Can you work these out from the drawing? Everything is in mm from the part's minimum corner. A direction names the side the tool comes from. Coordinates: 2 decimals unless noted, no trailing zeros. Loops run counter-clockwise (first coordinate to the right, second up) from the corner with the lowest first, then second, coordinate; pieces in that order, holes last. Notation, with made-up numbers: (54.5, -19.5) -> (108.5, -19.5) arc R11 ccw to (108.5, 1.5) -> close; hole circle Ø5 at (74.25, -35). An arc over 180 degrees is marked (long way). Use one line per item in the form item = value. Start each with the question number.
(1) I need wall thicknesses on line 1 (Z direction, x = 3, y = 24); line 2 (Z direction, x = 20.5, y = 12); line 3 (Y direction, x = 20.5, z = 23.5). Which ranges of each line are inside material? Lowest first, please. Write a range as [from, to].
(2) Imagine slicing it at A-A (y = 20). List the corners of the cut face in (x, z) for me, plus the area to 3 significant figures.
(3) I'm going to push flat-ended pins straight in: pin 1 (9 mm diameter, centred on x = 20, y = 20, fed in from +Z); pin 2 (6 mm diameter, centred on y = 23, z = 32.5, fed in from -X); pin 3 (3 mm diameter, centred on x = 3.5, y = 26, fed in from -Z). Where does each tip first touch, or does it pass through?
(4) On a 3-axis mill with a long thin cutter (end or side, diameter ignored), from which of +Z, -Z, +X, -X, +Y, -Y can I reach the whole of each face in a straight line? I mean the marked faces 1, 2 and 3. Say none if no direction works.
(5) Imagine slicing it at C-C (z = 37). List the corners of the cut face in (x, y) for me, plus the area to 3 significant figures.
(6) Imagine slicing it at B-B (x = 36). List the corners of the cut face in (y, z) for me.
(7) Imagine slicing it at D-D (y = 10). List the corners of the cut face in (x, z) for me, plus the area to 3 significant figures.
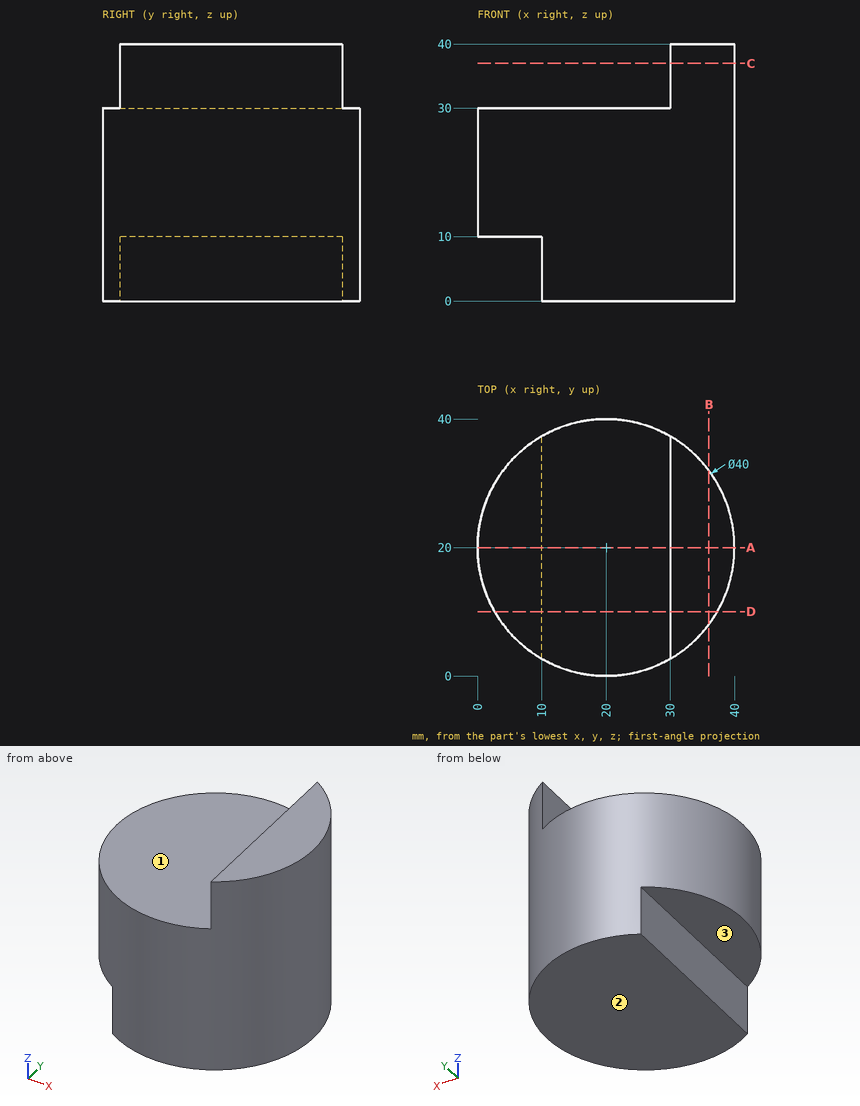
Worked out:
q1.line_1 = [10, 30]
q1.line_2 = [0, 30]
q1.line_3 = [0.01, 39.99]
q2.outline = (0, 10) -> (10, 10) -> (10, 0) -> (40, 0) -> (40, 40) -> (30, 40) -> (30, 30) -> (0, 30) -> close
q2.area = 1,200 mm2
q3.pin_1 = 30
q3.pin_2 = 0.05
q3.pin_3 = 10
q4.face_1 = +Z, -X, +Y, -Y
q4.face_2 = -Z, +X, -X, +Y, -Y
q4.face_3 = -Z, -X, +Y, -Y
q5.outline = (30, 2.68) arc R20 ccw to (30, 37.32) -> close
q5.area = 246 mm2
q6.outline = (8, 0) -> (32, 0) -> (32, 40) -> (8, 40) -> close
q7.outline = (2.68, 10) -> (10, 10) -> (10, 0) -> (37.32, 0) -> (37.32, 40) -> (30, 40) -> (30, 30) -> (2.68, 30) -> close
q7.area = 1,040 mm2
